The model under review builds one solid part; all positions refer to its coordinate system, in mm. Coordinates: 2 decimals unless noted, no trailing zeros. Order: outer loops, then holes, each group sorted by start corner. A loop starts at its lowest first (then second) coordinate and runs counter-clockwise, first axis right, second up. Notation, with made-up numbers: (-38, -8.75) -> (-18, -8.75) arc R28 cw to (-18, 24.25) -> close; hole circle Ø3 at (-33.75, 20). An arc over 180 degrees is marked (long way). Use one line per item in the form item = value. Start each with the question number.
(1) Take a section at C-C (z = 0.55). State how many separate pieces and enclosed holes the cut face has, then the cut area to 3 significant figures.
(2) Insertion check: pin 1 Ø2.5 at (x, z) = (80.5, 0) entering from +Y; pin 2 Ø2.5 at (y, z) = (68.5, -1) entering from -X; pin 3 Ø2.5 at (y, z) = (-6, -1) entering from +X. Each pin has a flat end and moves straight along its axis. Give the tip position at first contact, or say it passes through.
(3) Take a section at A-A (x = -89). State the section outline as (y, z) points.
(4) Take a section at D-D (x = 57). State the section outline as (y, z) points (1 decimal), then the cut area to 3 significant figures.
(5) Wall thickness on line 1 along X through (y, z) = (26.5, 1.05); line 2 along Y through (x, z) = (102, 0.9) (3 decimals); line 3 along X through (y, z) = (48, 0.75) (3 decimals): over which ranges is each line inside the solid? List them lowest first.
(6) Take a section at B-B (y = 95). State the section outline as (x, z) points, then the cut area to 3 significant figures.
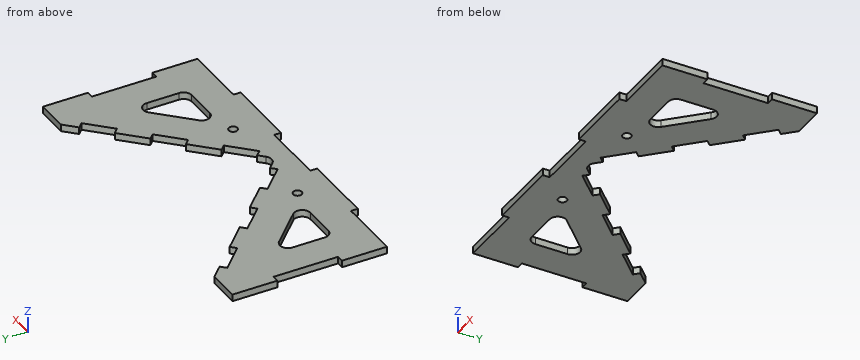
```python
from build123d import *

# Parameters (mm, degrees)
BOSS_EXTRUDE1_DEPTH     = 2.7305
CUT_EXTRUDE1_DEPTH      = 178.79882071
CAVITY1_START           = -133.35
CAVITY1_OUTLINE_W       = 50.8
CAVITY1_OUTLINE_H       = 5.461
CAVITY1_DEPTH           = 5.461
CAVITY1_START_2         = 127.889
CAVITY1_2_OUTLINE_W     = 50.8
CAVITY1_2_OUTLINE_H     = 5.461
CAVITY1_2_DEPTH         = 5.461
FILLET1_R               = 6.35
SKETCH3_W               = 5.461
SKETCH3_H               = 50.8
CUT_EXTRUDE2_DEPTH      = 178.79882071
FILLET2_R               = 6.35
F_1_4_CLEARANCE_HOLE1_D = 6.7564


# Read off the part's stored shape, not the designer's step: Cavity1
with BuildPart() as part:
    # Sketch1 → Boss-Extrude1 (new, symmetric)
    with BuildSketch(Plane.XY):
        Polygon((133.35, -4.064), (133.35, 117.475), (107.95, 117.475), (0, 9.525), (-107.95, 117.475), (-133.35, 117.475), (-133.35, -4.064), (-82.55, -4.064), (-82.55, -9.525), (-25.4, -9.525), (-25.4, -4.064), (25.4, -4.064), (25.4, -9.525), (82.55, -9.525), (82.55, -4.064), align=None)
    extrude(amount=BOSS_EXTRUDE1_DEPTH, both=True)

    # Sketch2 → Cut-Extrude1 (cut, through all)
    with BuildSketch(Plane.XY.offset(2.7305)):
        Polygon((-8.980256121, 18.505256121), (-12.841766253, 14.643745989), (-30.802278495, 32.604258231), (-26.940768363, 36.465768363), align=None)
        Polygon((-62.861792847, 72.386792847), (-66.72330298, 68.525282715), (-48.762790737, 50.564770473), (-44.901280605, 54.426280605), align=None)
        Polygon((-98.782817332, 108.307817332), (-102.644327464, 104.4463072), (-84.683815222, 86.485794958), (-80.82230509, 90.34730509), align=None)
        Polygon((80.82230509, 90.34730509), (98.782817332, 108.307817332), (102.644327464, 104.4463072), (84.683815222, 86.485794958), align=None)
        Polygon((44.901280605, 54.426280605), (62.861792847, 72.386792847), (66.72330298, 68.525282715), (48.762790737, 50.564770473), align=None)
        Polygon((26.940768363, 36.465768363), (30.802278495, 32.604258231), (12.841766253, 14.643745989), (8.980256121, 18.505256121), align=None)
    extrude(amount=-CUT_EXTRUDE1_DEPTH, mode=Mode.SUBTRACT)

    # Cavity1 outline → Cavity1 (cut)
    with BuildSketch(Plane.YZ.offset(CAVITY1_START)):
        with Locations((56.7055, 0)):
            Rectangle(CAVITY1_OUTLINE_W, CAVITY1_OUTLINE_H)
    extrude(amount=CAVITY1_DEPTH, mode=Mode.SUBTRACT)

    # Cavity1 2 outline → Cavity1 2 (cut)
    with BuildSketch(Plane.YZ.offset(CAVITY1_START_2)):
        with Locations((56.7055, 0)):
            Rectangle(CAVITY1_2_OUTLINE_W, CAVITY1_2_OUTLINE_H)
    extrude(amount=CAVITY1_2_DEPTH, mode=Mode.SUBTRACT)

    # Fillet1
    fillet1_edges = [part.edges().sort_by_distance(p)[0] for p in [
        (0, 9.525, 0),
    ]]
    fillet(fillet1_edges, radius=FILLET1_R)

    # Sketch3 → Cut-Extrude2 (cut, through all)
    with BuildSketch(Plane.XY.offset(2.7305)):
        with Locations((-130.6195, 56.7055)):
            Rectangle(SKETCH3_W, SKETCH3_H)
        Polygon((-102.489, 68.369955252), (-55.455044748, 21.336), (-102.489, 21.336), (-102.489, 31.3055), align=None)
    cut_extrude2 = extrude(amount=-CUT_EXTRUDE2_DEPTH, mode=Mode.SUBTRACT)

    # Mirror1: Cut-Extrude2 across plane
    add(cut_extrude2.mirror(Plane(origin=(0, 0, 0), x_dir=(0, 0, 1), z_dir=(1, 0, 0))), mode=Mode.SUBTRACT)

    # Fillet2
    fillet2_edges = [part.edges().sort_by_distance(p)[0] for p in [
        (-55.455044748, 21.336, 0),
        (-102.489, 21.336, 0),
        (-102.489, 68.369955252, 0),
        (102.489, 21.336, 0),
        (55.455044748, 21.336, 0),
        (102.489, 68.369955252, 0),
    ]]
    fillet(fillet2_edges, radius=FILLET2_R)

    # 1/4 Clearance Hole1 (through all)
    with Locations(Plane.XY.offset(2.7305)):
        with Locations((-45.327694765, 17.141114286)):
            f_1_4_clearance_hole1 = Hole(F_1_4_CLEARANCE_HOLE1_D / 2)

    # Mirror2: 1/4 Clearance Hole1 across plane
    add(f_1_4_clearance_hole1.mirror(Plane(origin=(0, 0, 0), x_dir=(0, 0, 1), z_dir=(1, 0, 0))), mode=Mode.SUBTRACT)


solid = part.part
```
Findings:
q1.separate_pieces = 1
q1.enclosed_holes = 4
q1.area = 17,900 mm²
q2.pin_1 = 90.35
q2.pin_2 = -127.89
q2.pin_3 = 82.55
q3.outline = (-4.06, -2.73) -> (21.34, -2.73) -> (21.34, 2.73) -> (-4.06, 2.73) -> close; (54.88, -2.73) -> (90.8, -2.73) -> (90.8, 2.73) -> (54.88, 2.73) -> close
q4.outline = (-9.5, -2.7) -> (58.8, -2.7) -> (58.8, 2.7) -> (-9.5, 2.7) -> close
q4.area = 373 mm²
q5.line_1 = -133.35 to -102.38, -64.55 to -24.7, 24.7 to 64.55, 102.38 to 133.35
q5.line_2 = -4.064 to 25.242, 55.483 to 103.802, 105.091 to 111.525
q5.line_3 = -127.889 to -102.489, -82.119 to -38.475, 38.475 to 82.119, 102.489 to 127.889
q6.outline = (-133.35, -2.73) -> (-93.2, -2.73) -> (-93.2, 2.73) -> (-133.35, 2.73) -> close; (93.2, -2.73) -> (133.35, -2.73) -> (133.35, 2.73) -> (93.2, 2.73) -> close
q6.area = 439 mm²
